Geometry: final body of the model. Coordinates: model frame, mm. Give positions to 0.01 mm unless a question says otherwise; leave off trailing zeros. Order: outer loops, then holes, each group sorted by start corner. A loop starts at its lowest first (then second) coordinate and runs counter-clockwise, first axis right, second up. Notation, with made-up numbers: (83.25, 59.5) - (131.25, 59.5) arc R18 ccw to (131.25, 79.5) - close; hole circle Ø11 at (80, 29). An arc over 180 degrees is marked (long way). One line per item, written item: value.
```python
from build123d import *

# Parameters (mm, degrees)
SKETCH1_R               = 9.5
SKETCH1_R_2             = 3.45
BOSS_EXTRUDE1_DEPTH     = 3.05
CUT_EXTRUDE1_DEPTH      = 15.754999153
CUT_EXTRUDE1_DEPTH_BACK = 15.754999153
SKETCH2_R               = 9.5
SKETCH2_R_2             = 9.2
CUT_EXTRUDE2_DEPTH      = 15.369759914
CUT_EXTRUDE2_DEPTH_BACK = 15.369759914
SKETCH3_R               = 3.7


with BuildPart() as part:
    # Sketch1 → Boss-Extrude1 (new, symmetric)
    with BuildSketch(Plane(origin=(0, 0, 0), x_dir=(1, 0, 0), z_dir=(0, 1, 0))):
        with Locations(Location((0, 0, 0), (0, 0, 270))):
            Circle(SKETCH1_R)
        with Locations(Location((0, 0, 0), (0, 0, 270))):
            Circle(SKETCH1_R_2, mode=Mode.SUBTRACT)
    extrude(amount=BOSS_EXTRUDE1_DEPTH, both=True)

    # Sketch2 → Cut-Extrude1 (cut, two sides: drawn at the far end of the back side and taken through both)
    with BuildSketch(Plane(origin=(0, 3.05, 0), x_dir=(1, 0, 0), z_dir=(0, 1, 0)).offset(-CUT_EXTRUDE1_DEPTH_BACK)):
        Circle(SKETCH2_R)
        with Locations(Location((0, 0, 0), (0, 0, 270))):
            Circle(SKETCH2_R_2, mode=Mode.SUBTRACT)
    extrude(amount=CUT_EXTRUDE1_DEPTH + CUT_EXTRUDE1_DEPTH_BACK, mode=Mode.SUBTRACT)

    # Sketch3 → Cut-Extrude2 (cut, two sides: drawn at the far end of the back side and taken through both)
    with BuildSketch(Plane(origin=(0, 3.05, 0), x_dir=(1, 0, 0), z_dir=(0, 1, 0)).offset(-CUT_EXTRUDE2_DEPTH_BACK)):
        with Locations(Location((0, 0, 0), (0, 0, 270))):
            Circle(SKETCH3_R)
    extrude(amount=CUT_EXTRUDE2_DEPTH + CUT_EXTRUDE2_DEPTH_BACK, mode=Mode.SUBTRACT)


solid = part.part
```
1) Mould query, pull axis X, two halves, no side actions, for faces 1 (the face through (-3.612, -0.043, -0.802)), 2 (the face through (0, 3.05, 4)), 3 (the face through (2.763, -0.043, 8.775)). Classes: released by +X, released by -X, zero draft, split by the parting line, or undercut.
Answers below:
face 1: undercut
face 2: zero draft
face 3: split by the parting line
2) Section D-D, the plane z = -8. Return loops of the section in (x, y).
Answers below:
outline: (-4.54, -3.05) - (4.54, -3.05) - (4.54, 3.05) - (-4.54, 3.05) - close
3) Section B-B, the plane x = 0. Return loops of the section in (y, z).
Answers below:
outline: (-3.05, -9.2) - (3.05, -9.2) - (3.05, -3.7) - (-3.05, -3.7) - close; (-3.05, 3.7) - (3.05, 3.7) - (3.05, 9.2) - (-3.05, 9.2) - close
4) Section A-A, the plane z = 0. Return loops of the section in (x, y).
Answers below:
outline: (-9.2, -3.05) - (-3.7, -3.05) - (-3.7, 3.05) - (-9.2, 3.05) - close; (3.7, -3.05) - (9.2, -3.05) - (9.2, 3.05) - (3.7, 3.05) - close
5) First-contact query: pin 1 (1 mm diameter, centred on y = -2, z = 3, fed in from -X); pin 2 (1 mm diameter, centred on y = 1, z = 0.5, fed in from -X); pin 3 (1.5 mm diameter, centred on x = -5, y = 0.5, fed in from -Z); pin 4 (6 mm diameter, centred on x = 0, z = 0, fed in from -Y). Flat tips, straight axial feed; report the tip coordinate or a pass-through.
Answers below:
pin 1: x = -8.85
pin 2: x = -9.2
pin 3: z = -8.16
pin 4: through
6) Section C-C, the plane y = -2. Return loops of the section in (x, z).
Answers below:
outline: circle Ø18.4 at (0, 0); hole circle Ø7.4 at (0, 0)
7) Material intervals for line 1 along X through (y, z) = (0.5, 0); line 2 along Z through (x, y) = (-0.75, -1.75), sorted ascending.
Answers below:
line 1: -9.2 to -3.7, 3.7 to 9.2
line 2: -9.17 to -3.62, 3.62 to 9.17
